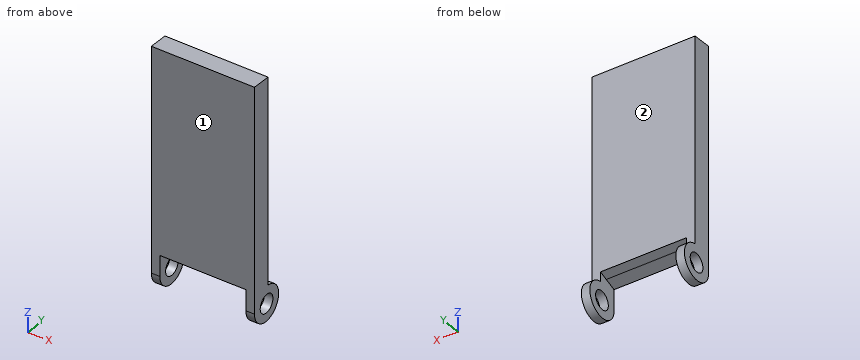
from build123d import *

# Parameters (mm, degrees)
SKETCH_1_W          = 20.2
SKETCH_1_H          = 30
EXTRUDE_1_DEPTH     = 2
SKETCH_2_R          = 4.2
SKETCH_2_R_2        = 2.2
EXTRUDE_2_DEPTH     = 2
EXTRUDE_3_DEPTH     = 2
CUT_EXTRUDE_1_REACH = 39.616
SKETCH_4_W          = 20.2
SKETCH_4_H          = 4
EXTRUDE_4_DEPTH     = 24.2
EXTRUDE_5_DEPTH     = 20.2
EXTRUDE_6_REACH     = 64.436
CUT_EXTRUDE_2_DEPTH = 20.2
CUT_EXTRUDE_3_REACH = 64.436


with BuildPart() as part:
    # 草图1 → 凸台-拉伸1 (new body)
    with BuildSketch(Plane(origin=(0, 0, 0), x_dir=(1, 0, 0), z_dir=(0, 1, 0))):
        with Locations((10.1, -15)):
            Rectangle(SKETCH_1_W, SKETCH_1_H)
    extrude(amount=EXTRUDE_1_DEPTH)

    # 草图2 → 凸台-拉伸2 (add)
    with BuildSketch(Plane.ZY):
        with Locations(Location((-2.5, 1.5, 0), (0, 0, 339.075167572))):
            Circle(SKETCH_2_R)
        with Locations((-2.5, 1.5)):
            Circle(SKETCH_2_R_2, mode=Mode.SUBTRACT)
    extrude_2 = extrude(amount=EXTRUDE_2_DEPTH)

    # 草图3 → 凸台-拉伸3 (add)
    with BuildSketch(Plane.ZY):
        with BuildLine():
            Line((1.423009049, 0), (30, 0))
            Line((30, 0), (30, 2))
            Line((30, 2), (1.670131892, 2))
            ThreePointArc((1.670131892, 2), (1.668300922, 0.984958812), (1.423009049, 0))
        make_face()
    extrude_3 = extrude(amount=EXTRUDE_3_DEPTH)

    # 镜向1: 凸台-拉伸2, 凸台-拉伸3 across plane
    add(extrude_2.mirror(Plane(origin=(10.1, 0, 0), x_dir=(0, 0, 1), z_dir=(1, 0, 0))))
    add(extrude_3.mirror(Plane(origin=(10.1, 0, 0), x_dir=(0, 0, 1), z_dir=(1, 0, 0))))

    # 草图4 → 切除-拉伸1 (cut, up to next)
    with BuildSketch(Plane(origin=(0, 2, 0), x_dir=(1, 0, 0), z_dir=(0, 1, 0)), mode=Mode.PRIVATE) as cut_extrude_1_sk1:
        with Locations((10.1, -2)):
            Rectangle(SKETCH_4_W, SKETCH_4_H)
    cut_extrude_1_tool1 = extrude(cut_extrude_1_sk1.sketch, amount=-CUT_EXTRUDE_1_REACH, mode=Mode.PRIVATE) & part.part
    add(cut_extrude_1_tool1.solids().sort_by_distance((10.1, 2, 2))[0], mode=Mode.SUBTRACT)

    # 草图7 → 凸台-拉伸4 (add)
    with BuildSketch(Plane.ZY.offset(2)):
        Polygon((30, 0), (56.65925637, 0), (57.272485309, 2), (30, 2), align=None)
    extrude(amount=-EXTRUDE_4_DEPTH)

    # 草图8 → 凸台-拉伸5 (add)
    with BuildSketch(Plane.ZY.offset(-20.2)):
        Polygon((4, 2), (3.386771061, 0), (4, 0), align=None)
    extrude(amount=EXTRUDE_5_DEPTH)

    # 凸台-拉伸6: up to this face of the body (flat: up to its plane)
    extrude_6_end = Plane(part.part.faces().sort_by_distance((22.2, 1.134069843, 20.823377478))[0])
    # 草图10 → 凸台-拉伸6 (add, up to the picked face)
    with BuildSketch(Plane.ZY.offset(2), mode=Mode.PRIVATE) as extrude_6_sk1:
        with BuildLine():
            Line((56.65925637, 0), (55.831397303, -2.7))
            Line((55.831397303, -2.7), (-2.5, -2.7))
            ThreePointArc((-2.5, -2.7), (-0.11882382, -1.959768778), (1.423009049, 0))
            Line((1.423009049, 0), (56.65925637, 0))
        make_face()
    extrude_6_tool1 = split(extrude(extrude_6_sk1.sketch, amount=-EXTRUDE_6_REACH, mode=Mode.PRIVATE), bisect_by=extrude_6_end, keep=Keep.BOTH, mode=Mode.PRIVATE)
    add(extrude_6_tool1.solids().sort_by(Axis((-2, -1.358557, 28.290322), (1, 0, 0)))[0])

    # 草图11 → 切除-拉伸2 (cut)
    with BuildSketch(Plane.ZY.offset(-20.2)):
        Polygon((3.386771061, 0), (2.558911994, -2.7), (-2.5, -2.7), (1.423009049, 0), align=None)
    extrude(amount=CUT_EXTRUDE_2_DEPTH, mode=Mode.SUBTRACT)

    # 草图15 → 切除-拉伸3 (cut, up to next)
    with BuildSketch(Plane.ZY.offset(2), mode=Mode.PRIVATE) as cut_extrude_3_sk1:
        Polygon((51.628649906, 2), (51.999830908, -2.7), (55.831397303, -2.7), (57.272485309, 2), align=None)
    cut_extrude_3_tool1 = extrude(cut_extrude_3_sk1.sketch, amount=-CUT_EXTRUDE_3_REACH, mode=Mode.PRIVATE) & part.part
    add(cut_extrude_3_tool1.solids().sort_by_distance((-2, -0.200179, 54.200143))[0], mode=Mode.SUBTRACT)


solid = part.part
Input: part model. Units: mm. Frame: model coordinates. Face numbers are marked on the shaded views. A direction names the side the tool comes from. Give positions to 0.01 mm unless a question says otherwise; leave off trailing zeros. Order: outer loops, then holes, each group sorted by start corner. A loop starts at its lowest first (then second) coordinate and runs counter-clockwise, first axis right, second up. Notation, with made-up numbers: (-6.5, -9) - (20.5, -9) arc R16 ccw to (20.5, -4) - close; hole circle Ø7 at (-12, 41). An arc over 180 degrees is marked (long way). Answer as a JSON object with one key per item and string values. Group by question number.
Q1. Set-up query: the marked faces 1 and 2. Return all of +Z, -Z, +X, -X, +Y, -Y with unobstructed straight access to the full face (end or side cutting, diameter ignored); none if empty.
Q2. Cut plane A-A, the plane y = 4.75. Output: boundary loops of the cut face in (x, z).
Q3. Cut plane C-C, the plane z = 28. Output: boundary loops of the cut face in (x, y).
Q4. Cut plane B-B, the plane x = 9.25. Output: boundary loops of the cut face in (y, z), then the cut area to 3 significant figures.
Q5. Line query: probe 1 along X at (y, z) = (2.75, 1); probe 2 along Y at (x, z) = (21.1, -2.5); probe 3 along Y at (x, z) = (7.5, 19). Output: solid intervals per line, ascending.
Q6. First-contact query: pin 1 Ø5 at (x, y) = (15.5, 4) entering from -Z; pin 2 Ø3 at (x, z) = (18.5, 27.5) entering from +Y; pin 3 Ø3 at (x, y) = (2.5, 2.5) entering from -Z; pin 4 Ø4 at (y, z) = (1.5, -2.5) entering from -X. Flat tips, straight axial feed; report the tip coordinate or a pass-through.
Results:
{
 "1": {"face 1": "+Z, -Z, +X, -X, -Y", "face 2": "+Z, +X, -X, +Y"},
 "2": {"outline": "(-2, -5.16) - (0, -5.16) - (0, 0.16) - (-2, 0.16) - close; (20.2, -5.16) - (22.2, -5.16) - (22.2, 0.16) - (20.2, 0.16) - close"},
 "3": {"outline": "(-2, -2.7) - (22.2, -2.7) - (22.2, 2) - (-2, 2) - close"},
 "4": {"outline": "(-2.7, 2.56) - (2, 4) - (2, 51.63) - (-2.7, 52) - close", "area": "228 mm^2"},
 "5": {"probe 1": "-2 to 0, 20.2 to 22.2", "probe 2": "-2.7 to -0.7, 3.7 to 5.7", "probe 3": "-2.7 to 2"},
 "6": {"pin 1": "z = 3.85", "pin 2": "y = 2", "pin 3": "z = 3.69", "pin 4": "through"}
}
